Model file for the job. Use its own axes, mm. Face numbers are marked on the shaded views. A direction names the side the tool comes from. Round coordinates to 2 decimals unless told otherwise and drop trailing zeros. Loops run counter-clockwise (first coordinate to the right, second up) from the corner with the lowest first, then second, coordinate; pieces in that order, holes last.
from build123d import *

# Parameters (mm, degrees)
BOSS_EXTRUDE1_DEPTH = 19.05
SKETCH3_W           = 77.47
SKETCH3_H           = 38.1
CUT_EXTRUDE1_DEPTH  = 2.54
CIRPATTERN1_COUNT   = 3
FILLET1_R           = 2.54


with BuildPart() as part:
    # Sketch1 → Boss-Extrude1 (new body, symmetric)
    with BuildSketch(Plane(origin=(0, 0, 0), x_dir=(1, 0, 0), z_dir=(0, 1, 0))):
        Polygon((0, 58.160560196), (-50.368522628, -29.080280098), (50.368522628, -29.080280098), align=None)
        Polygon((-39.37, -22.730280098), (39.37, -22.730280098), (0, 45.460560196), align=None, mode=Mode.SUBTRACT)
    extrude(amount=BOSS_EXTRUDE1_DEPTH, both=True)

    # Sketch3 → Cut-Extrude1 (cut)
    with BuildSketch(Plane.XY.offset(29.080280098)):
        Rectangle(SKETCH3_W, SKETCH3_H)
    cut_extrude1 = extrude(amount=-CUT_EXTRUDE1_DEPTH, mode=Mode.SUBTRACT)

    # CirPattern1: Cut-Extrude1 ×3 about axis
    cirpattern1_axis = Axis((0, 0, 0), (0, 1, 0))
    for i in range(1, CIRPATTERN1_COUNT):
        add(cut_extrude1.rotate(cirpattern1_axis, i * 360 / CIRPATTERN1_COUNT), mode=Mode.SUBTRACT)

    # Fillet1
    fillet1_edges = [part.edges().sort_by_distance(p)[0] for p in [
        (50.368522628, 0, 29.080280098),
        (-50.368522628, 0, 29.080280098),
        (0, 0, -58.160560196),
    ]]
    fillet(fillet1_edges, radius=FILLET1_R)


solid = part.part
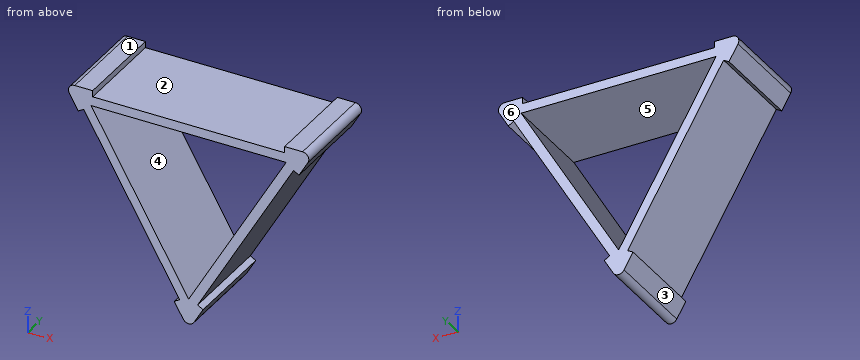
Q1. Slice it at A-A on y = -8. Give the cut face in (x, z) (3 decimals).
Q2. Slice it at B-B on x = -8.5. Give the cut face in (y, z), plus the area to 3 significant figures.
Q3. Pull direction X, two halves, no side cores. Call the marked faces 1, 2, 3 and 4: pulls with the +X half, pulls with the -X half, needs draft (parallel to the pull), parting line crosses it, or undercut.
Q4. Slice it at C-C on z = -28. Give the cut face in (x, y), plus the area to 3 significant figures.
Q5. Probe line 1 (X direction, y = -5.5, z = 20); line 2 (Z direction, x = -5, y = 14); line 3 (X direction, y = 14.5, z = -24.5). List the from-to ranges inside material, lowest first.
Q6. Flat gauge pins, fed straight in: P1, Ø8, axis at y = -9.5, z = 18.5, coming from the +X side; P2, Ø0.8, axis at y = -2, z = 27.5, coming from the +X side; P3, Ø12, axis at x = -26.5, y = -4.5, coming from the -Z side. Where does each tip first touch, or does it go through?
Q7. Tool access for the marked faces 5 and 6: list every direction of +Z, -Z, +X, -X, +Y, -Y with a clear straight run to the whole face (end or side of a thin tool).
Reply:
1. outline: (-48.169, 25.27) - (-44.552, 19.005) - (-42.352, 20.275) - (-3.617, -46.816) - (-5.817, -48.086) - (-2.2, -54.351) arc R2.54 ccw to (2.2, -54.351) - (5.817, -48.086) - (3.617, -46.816) - (42.352, 20.275) - (44.552, 19.005) - (48.169, 25.27) arc R2.54 ccw to (45.969, 29.08) - (38.735, 29.08) - (38.735, 26.54) - (-38.735, 26.54) - (-38.735, 29.08) - (-45.969, 29.08) arc R2.54 ccw to start; hole (-39.37, 22.73) - (0, -45.461) - (39.37, 22.73) - close
2. outline: (-19.05, -38.36) - (19.05, -38.36) - (19.05, -30.74) - (-19.05, -30.74) - close; (-19.05, 22.73) - (19.05, 22.73) - (19.05, 26.54) - (-19.05, 26.54) - close
2. area: 435 mm2
3. face 1: needs draft
3. face 2: undercut
3. face 3: pulls with the -X half
3. face 4: undercut
4. outline: (-14.48, -19.05) - (-10.08, -19.05) - (-10.08, 19.05) - (-14.48, 19.05) - close; (10.08, -19.05) - (14.48, -19.05) - (14.48, 19.05) - (10.08, 19.05) - close
4. area: 335 mm2
5. line 1: x = -45.13 to -42.83, -42.19 to -37.79, 37.79 to 42.19, 42.83 to 45.13
5. line 2: z = -49.5 to -47.61, -44.42 to -36.8, 22.73 to 26.54
5. line 3: x = -16.5 to -12.1, 12.1 to 16.5
6. P1: stops at x = 46.57
6. P2: stops at x = 48.45
6. P3: stops at z = -17.57
7. face 5: +Y, -Y
7. face 6: +Z, -Z, +X, -X, +Y
